from build123d import *

# Parameters (mm, degrees)
SKETCH1_R           = 28.1
BOSS_EXTRUDE1_DEPTH = 350
SKETCH2_R           = 18.6
CUT_EXTRUDE1_DEPTH  = 58.8
SKETCH3_W           = 222.683092022
SKETCH3_H           = 364.2827524
BOSS_EXTRUDE2_DEPTH = 58.8
SKETCH4_W           = 207.917403516
SKETCH4_H           = 348.54429772
CUT_EXTRUDE2_DEPTH  = 48.8
SKETCH5_R           = 16.1
CUT_EXTRUDE3_DEPTH  = 350
SKETCH6_R           = 3.75
CUT_EXTRUDE5_DEPTH  = 400
BOSS_EXTRUDE3_DEPTH = 10
SKETCH8_R           = 10
CUT_EXTRUDE7_DEPTH  = 10
SKETCH9_W           = 37.5
SKETCH9_H           = 1
BOSS_EXTRUDE4_DEPTH = 1
SKETCH10_W          = 37.5
SKETCH10_H          = 1
BOSS_EXTRUDE5_DEPTH = 1
SKETCH11_W          = 77.5
SKETCH11_H          = 1
BOSS_EXTRUDE6_DEPTH = 1
SKETCH12_W          = 77.5
SKETCH12_H          = 1
BOSS_EXTRUDE7_DEPTH = 1


with BuildPart() as part:
    # Sketch1 → Boss-Extrude1 (new body)
    with BuildSketch(Plane(origin=(0, 0, 0), x_dir=(1, 0, 0), z_dir=(0, 1, 0))):
        Circle(SKETCH1_R)
    extrude(amount=BOSS_EXTRUDE1_DEPTH)

    # Sketch2 → Cut-Extrude1 (cut)
    with BuildSketch(Plane(origin=(0, 350, 0), x_dir=(1, 0, 0), z_dir=(0, 1, 0))):
        with Locations((0, -7)):
            Circle(SKETCH2_R)
    extrude(amount=-CUT_EXTRUDE1_DEPTH, mode=Mode.SUBTRACT)

    # Sketch3 → Boss-Extrude2 (add)
    with BuildSketch(Plane(origin=(0, 0, 0), x_dir=(-1, 0, 0), z_dir=(0, -1, 0))):
        Rectangle(SKETCH3_W, SKETCH3_H)
    extrude(amount=BOSS_EXTRUDE2_DEPTH)

    # Sketch4 → Cut-Extrude2 (cut)
    with BuildSketch(Plane(origin=(0, -58.8, 0), x_dir=(-1, 0, 0), z_dir=(0, -1, 0))):
        Rectangle(SKETCH4_W, SKETCH4_H)
    extrude(amount=-CUT_EXTRUDE2_DEPTH, mode=Mode.SUBTRACT)

    # Sketch5 → Cut-Extrude3 (cut)
    with BuildSketch(Plane(origin=(0, 291.2, 0), x_dir=(1, 0, 0), z_dir=(0, 1, 0))):
        with Locations((0, -7)):
            Circle(SKETCH5_R)
    extrude(amount=-CUT_EXTRUDE3_DEPTH, mode=Mode.SUBTRACT)

    # Sketch6 → Cut-Extrude5 (cut)
    with BuildSketch(Plane(origin=(0, 350, 0), x_dir=(1, 0, 0), z_dir=(0, 1, 0))):
        with Locations((0, 18.75)):
            Circle(SKETCH6_R)
    extrude(amount=-CUT_EXTRUDE5_DEPTH, mode=Mode.SUBTRACT)

    # Sketch7 → Boss-Extrude3 (add)
    with BuildSketch(Plane(origin=(0, -10, 0), x_dir=(-1, 0, 0), z_dir=(0, -1, 0))):
        Polygon((-33, 69.189999926), (-30.5, 69.189999926), (-30.5, 146.689999926), (30.5, 146.689999926), (30.5, 109.189999926), (33, 109.189999926), (33, 149.189999926), (-33, 149.189999926), align=None)
    extrude(amount=BOSS_EXTRUDE3_DEPTH)

    # Sketch8 → Cut-Extrude7 (cut)
    with BuildSketch(Plane(origin=(0, 0, -182.1413762), x_dir=(-1, 0, 0), z_dir=(0, 0, -1))):
        with Locations((-86.573671766, -25.011155335)):
            Circle(SKETCH8_R)
    extrude(amount=-CUT_EXTRUDE7_DEPTH, mode=Mode.SUBTRACT)

    # Sketch9 → Boss-Extrude4 (add)
    with BuildSketch(Plane(origin=(-30.5, 0, 0), x_dir=(0, 0, -1), z_dir=(1, 0, 0))):
        with Locations((127.939999926, -19.5)):
            Rectangle(SKETCH9_W, SKETCH9_H)
    extrude(amount=BOSS_EXTRUDE4_DEPTH)

    # Sketch10 → Boss-Extrude5 (add)
    with BuildSketch(Plane(origin=(-30.5, 0, 0), x_dir=(0, 0, -1), z_dir=(1, 0, 0))):
        with Locations((127.939999926, -14.5)):
            Rectangle(SKETCH10_W, SKETCH10_H)
    extrude(amount=BOSS_EXTRUDE5_DEPTH)

    # Sketch11 → Boss-Extrude6 (add)
    with BuildSketch(Plane.ZY.offset(-30.5)):
        with Locations((-107.939999926, -19.5)):
            Rectangle(SKETCH11_W, SKETCH11_H)
    extrude(amount=BOSS_EXTRUDE6_DEPTH)

    # Sketch12 → Boss-Extrude7 (add)
    with BuildSketch(Plane.ZY.offset(-30.5)):
        with Locations((-107.939999926, -14.5)):
            Rectangle(SKETCH12_W, SKETCH12_H)
    extrude(amount=BOSS_EXTRUDE7_DEPTH)


solid = part.part
The model under review builds one solid part; all positions refer to its coordinate system, in mm. A direction names the side the tool comes from. Coordinates: 2 decimals unless noted, no trailing zeros. Loops run counter-clockwise (first coordinate to the right, second up) from the corner with the lowest first, then second, coordinate; pieces in that order, holes last. Notation, with made-up numbers: (81, 78) -> (91, 78) arc R19 ccw to (91, 97) -> close; hole circle Ø1 at (87.5, -12.5). An arc over 180 degrees is marked (long way). Use a Markdown table: item, result. Add a question column.
1. To check wall thickness, follow line 1 (Z direction, x = 0, y = 314); line 2 (Z direction, x = 0, y = 149); line 3 (Z direction, x = 51, y = -23). State the ranges of each line that lie inside material, in increasing order.
2. Machinability: for faces 1 (the face through (0, 350, -13)), 2 (the face through (33, -15, -110)), 3 (the face through (9.999, 321.012, -8.684)), which of the approach directions +Z, -Z, +X, -X, +Y, -Y give a long, thin tool a straight path to every point of the face, cutting with its end or side? Answer none if there is none.
3. Add section D-D on x = 9. Write out the cut boundary in (y, z), plus the area to 3 significant figures.
4. Add section A-A on z = 0. Write out the cut boundary in (x, y), plus the area to 3 significant figures.
5. Clearance check with flat-ended pins moving along their axes: pin 1 Ø10 at (x, z) = (-48, 35.5) entering from +Y; pin 2 Ø8 at (x, z) = (14, 22) entering from -Y; pin 3 Ø1.1 at (x, z) = (30, -111) entering from -Y. State where each tip first meets the part, or that it passes through.
6. Add section B-B on x = 60. Write out the cut boundary in (y, z).
7. Add section C-C on z = 119.5. Write out the cut boundary in (x, y), plus the area to 3 significant figures.
8. Draft analysis for pull direction Y (two halves, no side actions). For faces 4 (the face through (108, -58.8, -1)), 5 (the face through (2, 0, -43)), 6 (the face through (103.959, -35, 2)), 7 (the face through (88.741, -34.773, -178.262)), state which applies: pulls with the +Y half, pulls with the -Y half, needs draft (parallel to the pull), parting line crosses it, or undercut.
Returned:
| question | item | result |
|---|---|---|
| 1 | line 1 | z = -28.1 to -22.5, -15 to -11.6, 25.6 to 28.1 |
| 1 | line 2 | z = -28.1 to -22.5, -15 to -9.1, 23.1 to 28.1 |
| 1 | line 3 | z = -182.14 to -174.27, 174.27 to 182.14 |
| 2 | face 1 | +Z, -Z, +X, -X, +Y |
| 2 | face 2 | -Y |
| 2 | face 3 | +Y |
| 3 | outline | (-58.8, -182.14) -> (0, -182.14) -> (0, -26.62) -> (350, -26.62) -> (350, -9.28) -> (291.2, -9.28) -> (291.2, -6.35) -> (-10, -6.35) -> (-10, -146.69) -> (-20, -146.69) -> (-20, -149.19) -> (-10, -149.19) -> (-10, -174.27) -> (-58.8, -174.27) -> close; (-58.8, 174.27) -> (-10, 174.27) -> (-10, 20.35) -> (291.2, 20.35) -> (291.2, 23.28) -> (350, 23.28) -> (350, 26.62) -> (0, 26.62) -> (0, 182.14) -> (-58.8, 182.14) -> close |
| 3 | area | 13,100 mm² |
| 4 | outline | (-111.34, -58.8) -> (-103.96, -58.8) -> (-103.96, -10) -> (-14.5, -10) -> (-14.5, 291.2) -> (-17.23, 291.2) -> (-17.23, 350) -> (-28.1, 350) -> (-28.1, 0) -> (-111.34, 0) -> close; (14.5, -10) -> (103.96, -10) -> (103.96, -58.8) -> (111.34, -58.8) -> (111.34, 0) -> (28.1, 0) -> (28.1, 350) -> (17.23, 350) -> (17.23, 291.2) -> (14.5, 291.2) -> close |
| 4 | area | 11,900 mm² |
| 5 | pin 1 | stops at y = 0 |
| 5 | pin 2 | stops at y = -10 |
| 5 | pin 3 | stops at y = -20 |
| 6 | outline | (-58.8, -182.14) -> (0, -182.14) -> (0, 182.14) -> (-58.8, 182.14) -> (-58.8, 174.27) -> (-10, 174.27) -> (-10, -174.27) -> (-58.8, -174.27) -> close |
| 7 | outline | (-111.34, -58.8) -> (-103.96, -58.8) -> (-103.96, -10) -> (103.96, -10) -> (103.96, -58.8) -> (111.34, -58.8) -> (111.34, 0) -> (-111.34, 0) -> close |
| 7 | area | 2,950 mm² |
| 8 | face 4 | pulls with the -Y half |
| 8 | face 5 | pulls with the +Y half |
| 8 | face 6 | needs draft |
| 8 | face 7 | undercut |
